Can you work these out from the model? Positions are in its coordinate system, mm. Face numbers are marked on the shaded views. A direction names the side the tool comes from. Coordinates: 2 decimals unless noted, no trailing zeros. Order: outer loops, then holes, each group sorted by start corner. A loop starts at its lowest first (then second) coordinate and runs counter-clockwise, first axis right, second up. Notation, with made-up numbers: M 52.25,77 L 75.25,77 A17 cw 75.25,94 Z; hole C -37,-3 d11. An arc over 180 degrees is marked long. Answer as a JSON object with one key per item and string values.
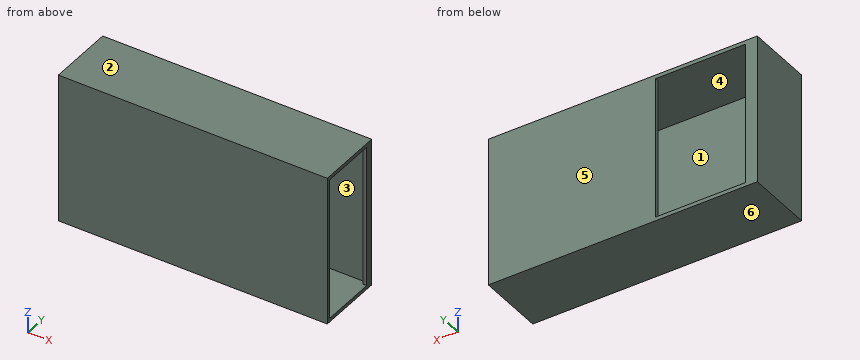
Autodesk Inventor part; units mm, degrees
ref_plane "YZ Plane" through (0, 0, 0) normal (1, 0, 0) x (0, 1, 0)
ref_plane "XZ Plane" through (0, 0, 0) normal (0, 1, 0) x (-1, 0, 0)
ref_plane "XY Plane" through (0, 0, 0) normal (0, 0, 1) x (1, 0, 0)
sketch "Sketch1" plane through (0, 0, 0) normal (0, 1, 0) x (-1, 0, 0)
  line L0 (0, 0) -> (-228.6, 0)
  line L1 (-228.6, 0) -> (-228.6, 127)
  line L2 (-228.6, 127) -> (0, 127)
  line L3 (0, 127) -> (0, 0)
  dimension "d0" = 228.6
  dimension "d1" = 127
extrude "Extrusion1" add sketch "Sketch1" along normal blind 3.175
sketch "Sketch2" plane through (0, 3.175, 0) normal (0, 1, 0) x (1, 0, 0)
  line L0 (228.6, 0) -> (0, 0)
  line L1 (0, -127) -> (228.6, -127)
  line L2 (0, 0) -> (228.6, 0)
  line L3 (228.6, -127) -> (0, -127)
  line L4 (0, -127) -> (0, 0)
  line L5 (0, 0) -> (0, -127)
  line L6 (0, 0) -> (228.6, 0)
  line L7 (228.6, 0) -> (228.6, -127)
  line L8 (228.6, -127) -> (0, -127)
  line L9 (0, -127) -> (0, 0)
  line L10 (228.6, -3.175) -> (3.175, -3.175)
  line L11 (3.175, -3.175) -> (3.175, -123.825)
  line L12 (3.175, -123.825) -> (228.6, -123.825)
  dimension "d4" = 3.175
extrude "Extrusion2" add sketch "Sketch2" along normal blind 50.8 contours L7 L10 L11 L12 L1 L4 L0
sketch "Sketch3" plane through (228.6, 0, 127) normal (1, 0, 0) x (0, 0, -1)
  line L0 (127, 53.975) -> (0, 53.975)
  line L1 (0, 53.975) -> (127, 53.975)
  line L2 (127, 53.975) -> (127, 0)
  line L3 (127, 0) -> (0, 0)
  line L4 (0, 0) -> (0, 53.975)
  line L5 (3.175, 50.8) -> (123.825, 50.8)
  line L6 (123.825, 50.8) -> (123.825, 3.175)
  line L7 (123.825, 3.175) -> (3.175, 3.175)
  line L8 (3.175, 3.175) -> (3.175, 50.8)
  dimension "d7" = 3.175
extrude "Extrusion3" add sketch "Sketch3" against normal blind 3.175
sketch "Sketch4" plane through (0, 53.975, 0) normal (0, 1, 0) x (1, 0, 0)
  line L0 (228.6, 0) -> (0, 0)
  line L1 (0, -127) -> (228.6, -127)
  line L2 (0, 0) -> (228.6, 0)
  line L3 (228.6, 0) -> (228.6, -127)
  line L4 (228.6, -127) -> (0, -127)
  line L5 (0, -127) -> (0, 0)
  line L6 (3.175, -123.825) -> (228.6, -123.825) construction
  line L7 (3.175, -123.825) -> (79.375, -123.825) construction
  line L8 (228.6, -127) -> (228.6, 0)
  line L9 (79.375, -123.825) -> (228.6, -123.825)
  line L10 (228.6, -123.825) -> (228.6, 0)
  line L11 (228.6, 0) -> (79.375, 0)
  line L12 (3.175, -123.825) -> (3.175, -3.175)
  line L13 (3.175, -3.175) -> (79.375, -3.175)
  line L14 (79.375, -123.825) -> (3.175, -123.825)
  line L15 (3.175, -123.825) -> (3.175, -3.175)
  line L16 (79.375, -3.175) -> (155.575, -3.175)
  line L17 (155.575, -123.825) -> (79.375, -123.825)
  line L18 (3.175, -123.825) -> (117.475, -123.825) construction
  line L19 (225.425, -123.825) -> (3.175, -123.825) construction
  line L20 (117.475, -123.825) -> (41.275, -123.825)
  line L21 (41.275, -3.175) -> (117.475, -3.175)
  line L22 (3.175, -3.175) -> (225.425, -3.175)
  line L23 (10.1575, -3.175) -> (86.3575, -3.175)
  line L24 (86.3575, -3.175) -> (86.3575, -123.825)
  line L25 (86.3575, -123.825) -> (10.1575, -123.825)
  line L26 (10.1575, -123.825) -> (10.1575, -3.175)
  point P0 (10.1575, -123.825)
  dimension "d10" = 76.2
  dimension "d13" = 76.2
  dimension "d15" = 114.3
  dimension "d16" = 76.2
  dimension "d17" = 76.2
extrude "Extrusion4" add sketch "Sketch4" along normal blind 3.175 contours L3 L1 L5 L0 | L14 L12 L13 L26
properties part number "ShootingMech_Housing3"
Item 1: I want a section at B-B, the plane x = 106.5. Write out the boundary of the cut face in (y, z) (3 decimals), plus the area to 3 significant figures.
Answers follow:
{"outline": "M 0,0 L 57.15,0 L 57.15,127 L 0,127 Z; hole M 3.175,3.175 L 53.975,3.175 L 53.975,123.825 L 3.175,123.825 Z", "area": "1,130 mm^2"}
Item 2: I'm going to push a flat-ended pin straight in: pin 1 (15 mm diameter, centred on y = 40, z = 73, fed in from +X) (3 decimals). Where does the tip first touch, or does it pass through?
Answers follow:
{"pin 1": "stops at x = 3.175"}
Item 3: If we mould it in two halves opening along Z, with no side actions, what happens to the marked faces 4, 5 and 6? For each: pulls with the +Z half, pulls with the -Z half, needs draft (parallel to the pull), parting line crosses it, or undercut.
Answers follow:
{"face 4": "undercut", "face 5": "needs draft", "face 6": "pulls with the -Z half"}
Item 4: Which directions (+Z, -Z, +X, -X, +Y, -Y) give clear straight access to the entire face, cutting with the end or side of a thin tool? Please do the marked faces 1, 2 and 3.
Answers follow:
{"face 1": "+X", "face 2": "+Z, +X, -X, +Y, -Y", "face 3": "none"}
Item 5: Please list where these lines run through material, in increasing order: line 1 (Z direction, x = 192.5, y = 24.5) (3 decimals); line 2 (Y direction, x = 145, z = 59) (3 decimals); line 3 (X direction, y = 52, z = 68.5) (3 decimals).
Answers follow:
{"line 1": "z = 0 to 3.175, 123.825 to 127", "line 2": "y = 0 to 3.175, 53.975 to 57.15", "line 3": "x = 0 to 3.175, 225.425 to 228.6"}
Item 6: I want a section at C-C, the plane y = 6.5. Write out the boundary of the cut face in (x, z) (3 decimals).
Answers follow:
{"outline": "M 0,0 L 228.6,0 L 228.6,3.175 L 3.175,3.175 L 3.175,123.825 L 228.6,123.825 L 228.6,127 L 0,127 Z"}
Item 7: I want a section at D-D, the plane x = 71. Write out the boundary of the cut face in (y, z) (3 decimals), plus the area to 3 significant figures.
Answers follow:
{"outline": "M 0,0 L 57.15,0 L 57.15,3.175 L 3.175,3.175 L 3.175,123.825 L 57.15,123.825 L 57.15,127 L 0,127 Z", "area": "746 mm^2"}
